from build123d import *

# Parameters (mm, degrees)
SKETCH1_W                   = 88
SKETCH1_H                   = 211
BOSS_EXTRUDE1_DEPTH         = 2
CUT_EXTRUDE2_DEPTH          = 2
SKETCH4_R                   = 5
CUT_EXTRUDE3_DEPTH          = 3
FILLET2_R                   = 3
BOSS_EXTRUDE2_DEPTH         = 10
CUT_EXTRUDE5_DEPTH          = 8
SKETCH58_R                  = 1.665
CUT_EXTRUDE9_DEPTH          = 1.8
SKETCH59_R                  = 2
CUT_EXTRUDE10_DEPTH         = 10
FILLET3_R                   = 0.5
F_3_0MM_DOWEL_HOLE1_D       = 3
TAP_DRILL_FOR_M3X0_5_TAP1_D = 2.5


with BuildPart() as part:
    # Sketch1 → Boss-Extrude1 (new body)
    with BuildSketch(Plane.XY):
        with Locations((44, 105.5)):
            Rectangle(SKETCH1_W, SKETCH1_H)
    extrude(amount=BOSS_EXTRUDE1_DEPTH)

    # Sketch3 → Cut-Extrude2 (cut)
    with BuildSketch(Plane.XY.offset(2)):
        Polygon((73, 115.5), (73, 133.88804004), (48, 148.32179677), (48, 115.5), align=None)
        Polygon((40, 148.32179677), (15, 133.88804004), (15, 115.5), (40, 115.5), align=None)
        Polygon((36, 155.25), (15, 167.374355653), (15, 143.125644347), align=None)
        Polygon((73, 143.125644347), (73, 167.374355653), (52, 155.25), align=None)
        Polygon((73, 196), (48, 196), (48, 162.17820323), (73, 176.61195996), align=None)
        Polygon((40, 196), (15, 196), (15, 176.61195996), (40, 162.17820323), align=None)
    cut_extrude2 = extrude(amount=-CUT_EXTRUDE2_DEPTH, mode=Mode.SUBTRACT)

    # Sketch4 → Cut-Extrude3 (cut, through all)
    with BuildSketch(Plane.XY.offset(2)):
        with Locations((44, 155.25)):
            Circle(SKETCH4_R)
    cut_extrude3 = extrude(amount=-CUT_EXTRUDE3_DEPTH, mode=Mode.SUBTRACT)

    # Mirror2: Cut-Extrude2, Cut-Extrude3 across plane
    add(cut_extrude2.mirror(Plane(origin=(0, 105.5, 0), x_dir=(0, 0, 1), z_dir=(0, -1, 0))), mode=Mode.SUBTRACT)
    add(cut_extrude3.mirror(Plane(origin=(0, 105.5, 0), x_dir=(0, 0, 1), z_dir=(0, -1, 0))), mode=Mode.SUBTRACT)

    # Fillet2
    fillet2_edges = [part.edges().sort_by_distance(p)[0] for p in [
        (36, 55.75, 1),
        (15, 43.625644347, 1),
        (15, 67.874355653, 1),
        (40, 95.5, 1),
        (40, 62.67820323, 1),
        (15, 77.11195996, 1),
        (15, 95.5, 1),
        (48, 48.82179677, 1),
        (73, 34.38804004, 1),
        (73, 15, 1),
        (48, 15, 1),
        (73, 43.625644347, 1),
        (52, 55.75, 1),
        (73, 67.874355653, 1),
        (15, 15, 1),
        (15, 34.38804004, 1),
        (40, 48.82179677, 1),
        (40, 15, 1),
        (73, 77.11195996, 1),
        (48, 62.67820323, 1),
        (48, 95.5, 1),
        (73, 95.5, 1),
        (15, 167.374355653, 1),
        (36, 155.25, 1),
        (15, 143.125644347, 1),
        (40, 148.32179677, 1),
        (40, 115.5, 1),
        (15, 115.5, 1),
        (15, 133.88804004, 1),
        (73, 176.61195996, 1),
        (48, 162.17820323, 1),
        (48, 196, 1),
        (73, 196, 1),
        (52, 155.25, 1),
        (73, 167.374355653, 1),
        (73, 143.125644347, 1),
        (15, 176.61195996, 1),
        (15, 196, 1),
        (40, 196, 1),
        (40, 162.17820323, 1),
        (48, 148.32179677, 1),
        (73, 133.88804004, 1),
        (73, 115.5, 1),
        (48, 115.5, 1),
    ]]
    fillet(fillet2_edges, radius=FILLET2_R)

    # Sketch7 → Boss-Extrude2 (add)
    with BuildSketch(Plane.XY.offset(2)):
        Polygon((94, 219), (84, 219), (84, 211), (88, 211), (88, 0), (84, 0), (84, -8), (94, -8), align=None)
        Polygon((-6, -8), (4, -8), (4, 0), (0, 0), (0, 211), (4, 211), (4, 219), (-6, 219), align=None)
    extrude(amount=-BOSS_EXTRUDE2_DEPTH)

    # Sketch53 → Cut-Extrude5 (cut)
    with BuildSketch(Plane(origin=(0, 0, -8), x_dir=(-1, 0, 0), z_dir=(0, 0, -1))):
        with BuildLine():
            Line((-90, 0), (-88, 0))
            Line((-88, 0), (-88, 211))
            Line((-88, 211), (-90, 211))
            ThreePointArc((-90, 211), (-91.414213562, 210.414213562), (-92, 209))
            Line((-92, 209), (-92, 2))
            ThreePointArc((-92, 2), (-91.414213562, 0.585786438), (-90, 0))
        make_face()
        with BuildLine():
            Line((2, 0), (-4, 0))
            Line((-4, 0), (-4, 211))
            Line((-4, 211), (2, 211))
            ThreePointArc((2, 211), (3.414213562, 210.414213562), (4, 209))
            Line((4, 209), (4, 2))
            ThreePointArc((4, 2), (3.414213562, 0.585786438), (2, 0))
        make_face()
    extrude(amount=-CUT_EXTRUDE5_DEPTH, mode=Mode.SUBTRACT)

    # Sketch58 → Cut-Extrude9 (cut)
    with BuildSketch(Plane(origin=(0, 0, 0), x_dir=(-1, 0, 0), z_dir=(0, 0, -1))):
        with Locations((-0.7, 13)):
            Circle(SKETCH58_R)
    cut_extrude9 = extrude(amount=-CUT_EXTRUDE9_DEPTH, mode=Mode.SUBTRACT)

    # Mirror4: Cut-Extrude9 across plane
    add(cut_extrude9.mirror(Plane(origin=(44, 0, 0), x_dir=(0, 0, 1), z_dir=(1, 0, 0))), mode=Mode.SUBTRACT)

    # Sketch59 → Cut-Extrude10 (cut)
    with BuildSketch(Plane(origin=(0, -8, 0), x_dir=(-1, 0, 0), z_dir=(0, -1, 0))):
        with Locations((-89, 2.4)):
            Circle(SKETCH59_R)
        with Locations((1, 2.4)):
            Circle(SKETCH59_R)
    extrude(amount=-CUT_EXTRUDE10_DEPTH, mode=Mode.SUBTRACT)

    # Fillet3
    fillet3_edges = [part.edges().sort_by_distance(p)[0] for p in [
        (94, 105.5, -8),
        (94, 105.5, 2),
        (-6, 105.5, -8),
        (-6, 105.5, 2),
    ]]
    fillet(fillet3_edges, radius=FILLET3_R)

    # Ø3.0mm Dowel Hole1 (through all)
    with Locations(Plane.XY.offset(2)):
        with Locations((24, 205), (64, 205), (9, 109.2), (79, 109.2), (9, 79.2), (79, 79.2), (9, 59.2), (79, 59.2), (9, 33.2), (79, 33.2), (13.7, 13), (24, 6), (74.3, 13), (64, 6)):
            Hole(F_3_0MM_DOWEL_HOLE1_D / 2)

    # Tap Drill for M3x0.5 Tap1 (through all)
    with Locations(Plane.XY.offset(2)):
        with Locations((9, 196), (79, 196), (9, 23), (79, 23)):
            Hole(TAP_DRILL_FOR_M3X0_5_TAP1_D / 2)


solid = part.part
Verification items for the finished model (mm, model axes). A direction names the side the tool comes from. Give positions to 0.01 mm unless a question says otherwise; leave off trailing zeros. Loops run counter-clockwise (first coordinate to the right, second up) from the corner with the lowest first, then second, coordinate; pieces in that order, holes last.
1. Release check for a two-part mould opening along Y. For faces 6 (the flat face through (4, -4, -3)), 7 (the flat face through (25.584, 49.736, 1.014)), 8 (the flat face through (89, 219, -3)) record: +Y half, -Y half, draft (parallel to the pull), parting line (faces both ways), or undercut.
Derived:
face 6: draft
face 7: undercut
face 8: +Y half
2. Material ranges on probe 1 along X at (y, z) = (205, 1.65); probe 2 along X at (y, z) = (98, -2); probe 3 along X at (y, z) = (109.2, 1.35), recorded low to high.
Derived:
probe 1: x = -5.98 to 22.5, 25.5 to 62.5, 65.5 to 93.98
probe 2: x = -6 to -4, 92 to 94
probe 3: x = -6 to 7.5, 10.5 to 77.5, 80.5 to 94
3. Tool access check on faces 1 (the flat face through (4, 215, -3)), 2 (the flat face through (61.867, 170.184, 1.014)), 3 (the flat face through (84, -4, -3)), 4 (the flat face through (-6, 107, -3)), 5 (the flat face through (-4, 107, -4)). Record the directions out of +Z, -Z, +X, -X, +Y, -Y that give a thin tool (end or side, any length) a straight path to the whole face; none if there is none.
Derived:
face 1: +Z, -Z, +Y
face 2: +Z, -Z
face 3: +Z, -Z, -Y
face 4: +Z, -Z, -X, +Y, -Y
face 5: -Z
4. Cross-section at A-A on y = 83. Record the cut outline in (x, z).
Derived:
outline: (-6, -7.5) arc R0.5 ccw to (-5.5, -8) - (-4, -8) - (-4, 0) - (15, 0) - (15, 2) - (-5.5, 2) arc R0.5 ccw to (-6, 1.5) - close; (40, 0) - (48, 0) - (48, 2) - (40, 2) - close; (73, 0) - (92, 0) - (92, -8) - (93.5, -8) arc R0.5 ccw to (94, -7.5) - (94, 1.5) arc R0.5 ccw to (93.5, 2) - (73, 2) - close
5. Go/stop test with flat-tipped pins: P1, Ø1.6, axis at x = 24.5, z = 0.5, coming from the -Y side; P2, Ø1.6, axis at x = 61, z = 1.5, coming from the +Y side; P3, Ø2.5, axis at x = 64, y = 6, coming from the +Z side; P4, Ø4, axis at x = 64, y = 205, coming from the -Z side. Record where each tip stops, or that it passes through.
Derived:
P1: stops at y = 0
P2: stops at y = 211
P3: passes through
P4: stops at z = 0
6. Cross-section at B-B on z = -2.4. Record the cut outline in (x, y), and give its area (3 significant figures).
Derived:
outline: (-6, -8) - (-3, -8) - (-3, 0.27) arc R2 cw to (-4, 2) - (-4, 209) arc R2 cw to (-2, 211) - (4, 211) - (4, 219) - (-6, 219) - close; (1, -8) - (4, -8) - (4, 0) - (1, 0) - close; (84, -8) - (87, -8) - (87, 0) - (84, 0) - close; (84, 211) - (90, 211) arc R2 cw to (92, 209) - (92, 2) arc R2 cw to (91, 0.27) - (91, -8) - (94, -8) - (94, 219) - (84, 219) - close
area: 1,100 mm2
